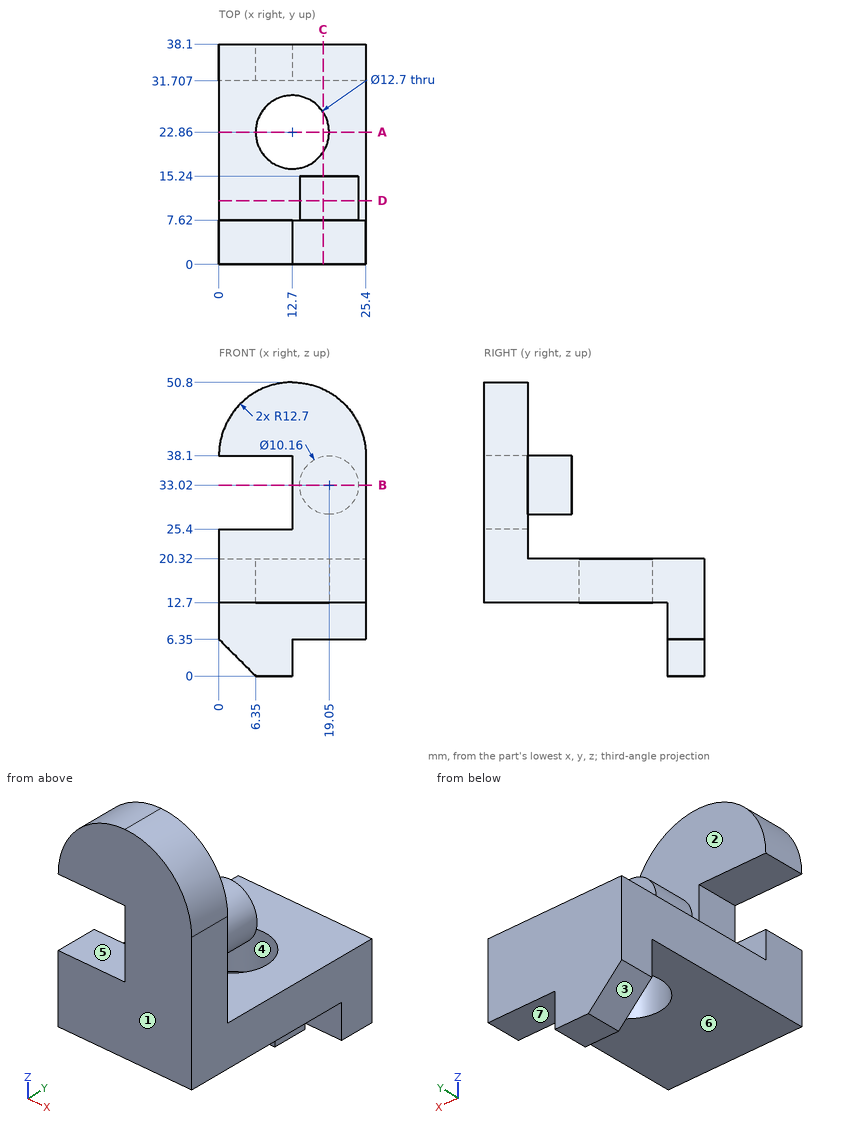
Input: dimensioned drawing with shaded views. Units: mm. Origin: part minimum x, y, z. A direction names the side the tool comes from. Round coordinates to 2 decimals unless told otherwise and drop trailing zeros. Order: outer loops, then holes, each group sorted by start corner. A loop starts at its lowest first (then second) coordinate and runs counter-clockwise, first axis right, second up.
Q1. Pin query (flat end, axial travel): pin 1 (12.5 mm diameter, centred on x = 9, y = 19.5, fed in from +Z); pin 2 (10 mm diameter, centred on x = 12.7, y = 22.86, fed in from -Z); pin 3 (1.5 mm diameter, centred on x = 13, y = 11.5, fed in from -Z); pin 4 (1 mm diameter, centred on x = 16.5, y = 14, fed in from +Z). Return the tip coordinate at first contact, or that it passes through.
Result sheet:
pin 1: stops at z = 20.32
pin 2: passes through
pin 3: stops at z = 12.7
pin 4: stops at z = 37.67
Q2. Mould query, pull axis Y, two halves, no side actions, for the marked faces 1, 2, 3 and 4. Classes: released by +Y, released by -Y, zero draft, split by the parting line, or undercut.
Result sheet:
face 1: released by -Y
face 2: released by +Y
face 3: zero draft
face 4: undercut
Q3. Material intervals for probe 1 along Y at (x, z) = (12.7, 18.5); probe 2 along Z at (x, y) = (3.75, 7.5); probe 3 along Y at (x, z) = (4.5, 24.5), sorted ascending.
Result sheet:
probe 1: y = 0 to 16.51, 29.21 to 38.1
probe 2: z = 12.7 to 25.4, 38.1 to 47.11
probe 3: y = 0 to 7.62
Q4. Section D-D, the plane y = 11. Output: boundary loops of the cut face in (x, z).
Result sheet:
outline: (0, 12.7) - (25.4, 12.7) - (25.4, 20.32) - (0, 20.32) - close; circle Ø10.16 at (19.05, 33.02)
Q5. Section B-B, the plane z = 33.02. Output: boundary loops of the cut face in (x, y).
Result sheet:
outline: (12.7, 0) - (25.4, 0) - (25.4, 7.62) - (24.13, 7.62) - (24.13, 15.24) - (13.97, 15.24) - (13.97, 7.62) - (12.7, 7.62) - close
Q6. Section A-A, the plane y = 22.86. Output: boundary loops of the cut face in (x, z).
Result sheet:
outline: (0, 12.7) - (6.35, 12.7) - (6.35, 20.32) - (0, 20.32) - close; (19.05, 12.7) - (25.4, 12.7) - (25.4, 20.32) - (19.05, 20.32) - close
Q7. Section C-C, the plane x = 18. Output: boundary loops of the cut face in (y, z), and give its area (3 significant figures).
Result sheet:
outline: (0, 12.7) - (19.36, 12.7) - (19.36, 20.32) - (7.62, 20.32) - (7.62, 28.05) - (15.24, 28.05) - (15.24, 37.99) - (7.62, 37.99) - (7.62, 49.64) - (0, 49.64) - close; (26.36, 12.7) - (31.71, 12.7) - (31.71, 6.35) - (38.1, 6.35) - (38.1, 20.32) - (26.36, 20.32) - close
area: 577 mm2
Q8. Access query for the marked faces 5, 6 and 7. Directions: +Z, -Z, +X, -X, +Y, -Y. A direction counts if a zero-diameter tool reaches every point of the face in a straight line with its end or side. Return the directions, or none.
Result sheet:
face 5: -X, +Y, -Y
face 6: -Z, +X, -X, -Y
face 7: -Z, +X, +Y, -Y
